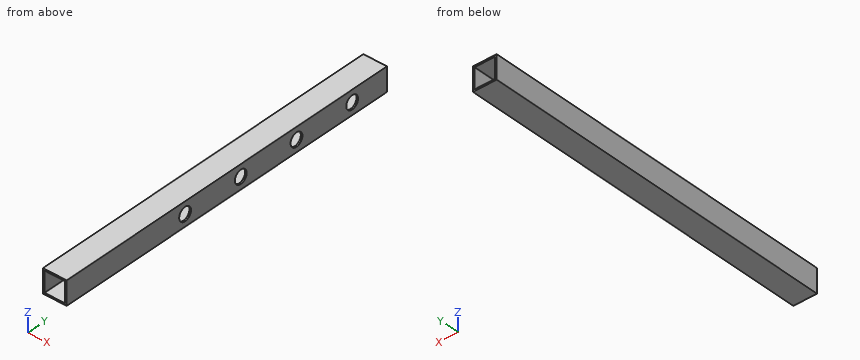
Autodesk Inventor part; units mm, degrees
ref_plane "YZ Plane" through (0, 0, 0) normal (1, 0, 0) x (0, 1, 0)
ref_plane "XZ Plane" through (0, 0, 0) normal (0, 1, 0) x (-1, 0, 0)
ref_plane "XY Plane" through (0, 0, 0) normal (0, 0, 1) x (1, 0, 0)
sketch "Sketch9" plane through (0, 0, 0) normal (0, 1, 0) x (-1, 0, 0)
  line L0 (15, 15) -> (-15, 15)
  line L1 (-15, 15) -> (-15, -15)
  line L2 (-15, -15) -> (15, -15)
  line L3 (15, -15) -> (15, 15)
  line L4 (15, 15) -> (-15, -15) construction
  line L5 (-15, 15) -> (15, -15) construction
  line L6 (-13, 13) -> (13, 13)
  line L7 (13, 13) -> (13, -13)
  line L8 (13, -13) -> (-13, -13)
  line L9 (-13, -13) -> (-13, 13)
  point P0 (0, 0)
  dimension "d172" = 30
  dimension "d173" = 30
  dimension "d174" = 2
extrude "Extrusion3" add sketch "Sketch9" against normal blind 460
sketch "Sketch10" plane through (0, 0, 0) normal (1, 0, 0) x (0, 1, 0)
  line L0 (0, 15) -> (0, -15) construction
  line L1 (0, 15) -> (-460, 15) construction
  line L2 (0, -15) -> (-460, -15) construction
  line L3 (-58.5, 8.5) -> (-41.5, 8.5)
  line L4 (-41.5, 8.5) -> (-41.5, -8.5)
  line L5 (-41.5, -8.5) -> (-58.5, -8.5)
  line L6 (-58.5, -8.5) -> (-58.5, 8.5)
  line L7 (-58.5, 8.5) -> (-41.5, -8.5) construction
  line L8 (-41.5, 8.5) -> (-58.5, -8.5) construction
  line L9 (0, 0) -> (30, 0)
  circle A0 centre (-50, 0) radius 8.5
  dimension "d177" = 17
  dimension "d178" = 17
  dimension "d181" = 30
  dimension "d182" = 80
extrude "Extrusion4" cut sketch "Sketch10" along normal through all contours A0
pattern_linear "Rectangular Pattern4" count 4 spacing 80 along (0, -1, 0) of "Extrusion4"
properties part number "PRS 1662 DrSysB way tube 2_1200" material "Stainless Steel"
Source: CAD feature listing. Evaluate the final solid. Frame: model axes, mm. Coordinates: 2 decimals unless noted, no trailing zeros. Write each loop counter-clockwise with the first axis right and the second up, starting at its lowest first coordinate (ties: lowest second). Pieces come first, ordered by that corner, then holes. Notation, with made-up numbers: (46.25, 60) -> (69.25, 60) arc R21 ccw to (69.25, 64) -> close; hole circle Ø11 at (19.25, 64). An arc over 180 degrees is marked (long way). Return JSON: item names as keys, results as strings. Group by question number.
1) Section query C-C, the plane y = -321. Return loops of the section in (x, z).
2) Contact query for a flat-ended pin moving along its axis: P1, Ø1, axis at y = -213.5, z = -6.5, coming from the +X side. Output: stop coordinate, or through.
3) Section query A-A, the plane x = -2. Return loops of the section in (y, z).
4) Section query B-B, the plane z = 0. Return loops of the section in (x, y).
5) Section query D-D, the plane y = -210. Return loops of the section in (x, z).
6) Ray query, line 1 along Y through (x, z) = (13.9, 0); line 2 along Z through (x, y) = (6.75, -426.5); line 3 along Z through (x, y) = (14.05, -290). Return the intervals inside material, ascending.
From the geometry:
{
 "1": {"outline": "(-15, -15) -> (15, -15) -> (15, 15) -> (-15, 15) -> close; hole (-13, -13) -> (13, -13) -> (13, 13) -> (-13, 13) -> close"},
 "2": {"P1": "x = -13"},
 "3": {"outline": "(-460, -15) -> (0, -15) -> (0, -13) -> (-460, -13) -> close; (-460, 13) -> (0, 13) -> (0, 15) -> (-460, 15) -> close"},
 "4": {"outline": "(-15, -460) -> (-13, -460) -> (-13, 0) -> (-15, 0) -> close; (13, -460) -> (15, -460) -> (15, -298.5) -> (13, -298.5) -> close; (13, -281.5) -> (15, -281.5) -> (15, -218.5) -> (13, -218.5) -> close; (13, -201.5) -> (15, -201.5) -> (15, -138.5) -> (13, -138.5) -> close; (13, -121.5) -> (15, -121.5) -> (15, -58.5) -> (13, -58.5) -> close; (13, -41.5) -> (15, -41.5) -> (15, 0) -> (13, 0) -> close"},
 "5": {"outline": "(-15, -15) -> (15, -15) -> (15, -8.5) -> (13, -8.5) -> (13, -13) -> (-13, -13) -> (-13, 13) -> (13, 13) -> (13, 8.5) -> (15, 8.5) -> (15, 15) -> (-15, 15) -> close"},
 "6": {"line 1": "-460 to -298.5, -281.5 to -218.5, -201.5 to -138.5, -121.5 to -58.5, -41.5 to 0", "line 2": "-15 to -13, 13 to 15", "line 3": "-15 to -8.5, 8.5 to 15"}
}
